```python
from build123d import *

# Parameters (mm, degrees)
MINOR_FILLET_SMOOTHING_R = 0.127


with BuildPart() as part:
    # Sketch1 → Revolve1 (revolve)
    with BuildSketch(Plane(origin=(0, 0, 0), x_dir=(1, 0, 0), z_dir=(0, 1, 0))):
        Polygon((6.885, -6.35), (9.525, -6.35), (9.525, 0), (11.1125, 0), (11.1125, 3.175), (6.885, 3.175), align=None)
    revolve(axis=Axis((0, 0, -3.175), (0, 0, 1)))

    # Minor Fillet Smoothing
    minor_fillet_smoothing_edges = [part.edges().sort_by_distance(p)[0] for p in [
        (-11.1125, 0, -3.175),
        (-11.1125, 0, 0),
        (-9.525, 0, 0),
        (-9.525, 0, 6.35),
    ]]
    fillet(minor_fillet_smoothing_edges, radius=MINOR_FILLET_SMOOTHING_R)


solid = part.part
```
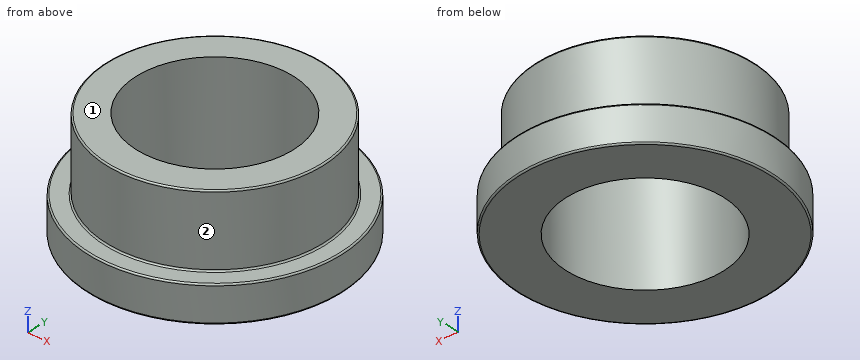
Can you work these out from the model? Positions are in its coordinate system, mm. Face numbers are marked on the shaded views. A direction names the side the tool comes from. Coordinates: 2 decimals unless noted, no trailing zeros. Write each loop counter-clockwise with the first axis right and the second up, starting at its lowest first coordinate (ties: lowest second). Pieces come first, ordered by that corner, then holes. Notation, with made-up numbers: (43.5, -24) - (97.5, -24) arc R28 cw to (97.5, 5) - close; hole circle Ø5 at (3.25, 75). An arc over 180 degrees is marked (long way). Return JSON: item names as keys, results as strings.
Q1. If we section it at C-C (z = 4): Please give me the cut outline in (x, y) (3 decimals).
Computed values:
{"outline": "circle Ø19.05 at (0, 0); hole circle Ø13.77 at (0, 0)"}
Q2. On a 3-axis mill with a long thin cutter (end or side, diameter ignored), from which of +Z, -Z, +X, -X, +Y, -Y can I reach the whole of each face in a straight line? I mean the marked faces 1 and 2. Say none if no direction works.
Computed values:
{"face 1": "+Z, +X, -X, +Y, -Y", "face 2": "+Z"}
Q3. Please list where these lines run through material, in increasing order: L1, parallel to Y at x = 0, z = 1 (3 decimals); L2, parallel to X at y = 5, z = -0.75; L3, parallel to X at y = 4.75, z = -2. Write a range as from..to.
Computed values:
{"L1": "y = -9.525..-6.885, 6.885..9.525", "L2": "x = -9.92..-4.73, 4.73..9.92", "L3": "x = -10.05..-4.98, 4.98..10.05"}
Q4. If we section it at D-D (z = -1.75): Please give me the cut outline in (x, y) (1 decimal), then the cut area to 3 significant figures.
Computed values:
{"outline": "circle Ø22.2 at (0, 0); hole circle Ø13.8 at (0, 0)", "area": "239 mm2"}
Q5. I'm going to push flat-ended pins straight in: pin 1 Ø1 at (x, z) = (3, 5) entering from +Y; pin 2 Ø3 at (x, z) = (-2.5, 5) entering from -Y; pin 3 Ø1.5 at (y, z) = (6.5, 0.5) entering from -X; pin 4 Ø6 at (x, y) = (8.5, 5.5) entering from +Z. Where does each tip first touch, or does it pass through?
Computed values:
{"pin 1": "stops at y = 9.19", "pin 2": "stops at y = -9.47", "pin 3": "stops at x = -9.33", "pin 4": "stops at z = 6.35"}
